Verification items for the finished model (mm, model axes). A direction names the side the tool comes from. Give positions to 0.01 mm unless a question says otherwise; leave off trailing zeros. Write each loop counter-clockwise with the first axis right and the second up, starting at its lowest first coordinate (ties: lowest second). Pieces come first, ordered by that corner, then holes.
Autodesk Inventor part; units mm, degrees
ref_plane "YZ Plane" through (0, 0, 0) normal (1, 0, 0) x (0, 1, 0)
ref_plane "XZ Plane" through (0, 0, 0) normal (0, 1, 0) x (-1, 0, 0)
ref_plane "XY Plane" through (0, 0, 0) normal (0, 0, 1) x (1, 0, 0)
sketch "Sketch1" plane through (0, 0, 0) normal (0, 0, 1) x (1, 0, 0)
  circle A0 centre (0, 0) radius 28.575
  dimension "d0" = 57.15
extrude "Extrusion1" add sketch "Sketch1" along normal blind 28.575
sketch "Sketch2" plane through (0, 0, 28.575) normal (0, 0, 1) x (1, 0, 0)
  circle A0 centre (0, 0) radius 28.575
  circle A1 centre (0, 0) radius 26.035
  dimension "d4" = 52.07
extrude "Extrusion2" cut sketch "Sketch2" against normal blind 1.27 contours A1
fillet "Fillet1" radius 3.175 1 edges at (-28.575, 0, 0)
properties part number "Lg Motor Bottom" material "ABS Plastic"
Item 1: Sectioned sample at A-A on x = 0. Record the cut outline in (y, z) (3 decimals).
Answer key:
outline: (-28.575, 3.175) arc R3.175 ccw to (-25.4, 0) - (25.4, 0) arc R3.175 ccw to (28.575, 3.175) - (28.575, 28.575) - (26.035, 28.575) - (26.035, 27.305) - (-26.035, 27.305) - (-26.035, 28.575) - (-28.575, 28.575) - close
Item 2: Set-up check for faces 1 (the face through (13, -23, 28.575)), 2 (the face through (0, 0, 27.305)): record each of +Z, -Z, +X, -X, +Y, -Y from which the full face is reachable in a straight line by a thin tool's end or side.
Answer key:
face 1: +Z, +X, -X, +Y, -Y
face 2: +Z
Item 3: Depth check by flat-ended pin: pin 1 (12 mm diameter, centred on y = -16.5, z = 18.5, fed in from +X); pin 2 (1 mm diameter, centred on x = -3.5, z = 7, fed in from -Y); pin 3 (10 mm diameter, centred on x = -0.5, z = 18, fed in from +Y) (3 decimals). Enter the tip coordinate at first touch or a pass-through.
Answer key:
pin 1: stops at x = 26.58
pin 2: stops at y = -28.42
pin 3: stops at y = 28.575
Item 4: Sectioned sample at C-C on z = 9.5. Record the cut outline in (x, y) (3 decimals).
Answer key:
outline: circle Ø57.15 at (0, 0)
Item 5: Release check for a two-part mould opening along Y. For faces 3 (the face through (-28.547, -1.256, 15.697)), 4 (the face through (-3.389, 25.813, 27.949)), 5 (the face through (0, 0, 0)) record: released by +Y, released by -Y, zero draft, split by the parting line, or undercut.
Answer key:
face 3: split by the parting line
face 4: undercut
face 5: zero draft
Item 6: Scan lines: line 1 along Y through (x, z) = (0, 27.85) (3 decimals); line 2 along Z through (x, y) = (-8, 21) (3 decimals); line 3 along Y through (x, z) = (-21, 3). Record each from-to range of solid material in increasing order.
Answer key:
line 1: y = -28.575 to -26.035, 26.035 to 28.575
line 2: z = 0 to 27.305
line 3: y = -19.37 to 19.37
